from build123d import *

# Parameters (mm, degrees)
SKETCH1_W           = 25.4
SKETCH1_H           = 25.4
BOSS_EXTRUDE1_DEPTH = 533.4
SHELL1_T            = -1.5875
SKETCH3_R           = 2.4892
CUT_EXTRUDE1_DEPTH  = 533.4
SKETCH4_R           = 2.4892
CUT_EXTRUDE2_DEPTH  = 533.4


with BuildPart() as part:
    # Sketch1 → Boss-Extrude1 (new, symmetric)
    with BuildSketch(Plane.XY):
        with Locations((12.7, 12.7)):
            Rectangle(SKETCH1_W, SKETCH1_H)
    extrude(amount=BOSS_EXTRUDE1_DEPTH, both=True)

    # Shell1
    shell1_openings = [part.faces().sort_by_distance(p)[0] for p in [
        (12.7, 12.7, 533.4),
        (12.7, 12.7, -533.4),
    ]]
    offset(amount=SHELL1_T, openings=shell1_openings, kind=Kind.INTERSECTION)

    # Sketch3 → Cut-Extrude1 (cut, symmetric)
    with BuildSketch(Plane(origin=(0, 25.4, 0), x_dir=(1, 0, 0), z_dir=(0, 1, 0))):
        with Locations(Location((12.7, -520.7, 0), (0, 0, 90))):
            Circle(SKETCH3_R)
        with Locations(Location((12.7, -495.3, 0), (0, 0, 90))):
            Circle(SKETCH3_R)
        with Locations(Location((12.7, -469.9, 0), (0, 0, 90))):
            Circle(SKETCH3_R)
    cut_extrude1 = extrude(amount=CUT_EXTRUDE1_DEPTH, both=True, mode=Mode.SUBTRACT)

    # Sketch4 → Cut-Extrude2 (cut, symmetric)
    with BuildSketch(Plane.ZY):
        with Locations((520.7, 12.7)):
            Circle(SKETCH4_R)
        with Locations((495.3, 12.7)):
            Circle(SKETCH4_R)
        with Locations((469.9, 12.7)):
            Circle(SKETCH4_R)
    cut_extrude2 = extrude(amount=CUT_EXTRUDE2_DEPTH, both=True, mode=Mode.SUBTRACT)

    # Mirror1: Cut-Extrude1, Cut-Extrude2 across plane
    add(cut_extrude1.mirror(Plane.XY), mode=Mode.SUBTRACT)
    add(cut_extrude2.mirror(Plane.XY), mode=Mode.SUBTRACT)


solid = part.part
The model under review builds one solid part; all positions refer to its coordinate system, in mm. A direction names the side the tool comes from. Round coordinates to 2 decimals unless told otherwise and drop trailing zeros. Loops run counter-clockwise (first coordinate to the right, second up) from the corner with the lowest first, then second, coordinate; pieces in that order, holes last. Notation, with made-up numbers: (-36, -15.75) - (-22, -15.75) arc R15 ccw to (-22, -8.75) - close; hole circle Ø6 at (-12, 70). An arc over 180 degrees is marked (long way). Use CSV: the item, a comma, the result in double quotes.
(1) The part is to be moulded in two halves that separate along X. For faces 1 (the flat face through (13, 1.588, 7)), 2 (the flat face through (0, 13, 7)), 3 (the flat face through (1, 13, 533.4)), say which applies: pulls with the +X half, pulls with the -X half, needs draft (parallel to the pull), parting line crosses it, or undercut.
Working result:
face 1,"undercut"
face 2,"pulls with the -X half"
face 3,"needs draft"
(2) Clearance check with a flat-ended pin moving along its axis: P1, Ø8, axis at x = 6.5, y = 19, coming from the +Z side. State where the tip first meets the part, or that it passes through.
Working result:
P1,"passes through"
(3) Take a section at A-A, the plane z = -64. Give the boundary of the cut face in (x, y).
Working result:
outline,"(0, 0) - (25.4, 0) - (25.4, 25.4) - (0, 25.4) - close; hole (1.59, 1.59) - (23.81, 1.59) - (23.81, 23.81) - (1.59, 23.81) - close"
(4) For line 1 (Y direction, x = 13.25, z = -415); line 2 (Y direction, x = 1, z = 495.3), list the stretches that pass through material, from the lowest coordinate up.
Working result:
line 1,"y = 0 to 1.59, 23.81 to 25.4"
line 2,"y = 0 to 10.21, 15.19 to 25.4"
(5) Take a section at B-B, the plane x = 5.75. Give the boundary of the cut face in (y, z).
Working result:
outline,"(0, -533.4) - (1.59, -533.4) - (1.59, 533.4) - (0, 533.4) - close; (23.81, -533.4) - (25.4, -533.4) - (25.4, 533.4) - (23.81, 533.4) - close"
(6) Machinability: for faces 4 (the flat face through (13, 0, 7)), 5 (the flat face through (1.588, 13, 7)), which of the approach directions +Z, -Z, +X, -X, +Y, -Y give a long, thin tool a straight path to every point of the face, cutting with its end or side? Answer none if there is none.
Working result:
face 4,"+Z, -Z, +X, -X, -Y"
face 5,"+Z, -Z"
